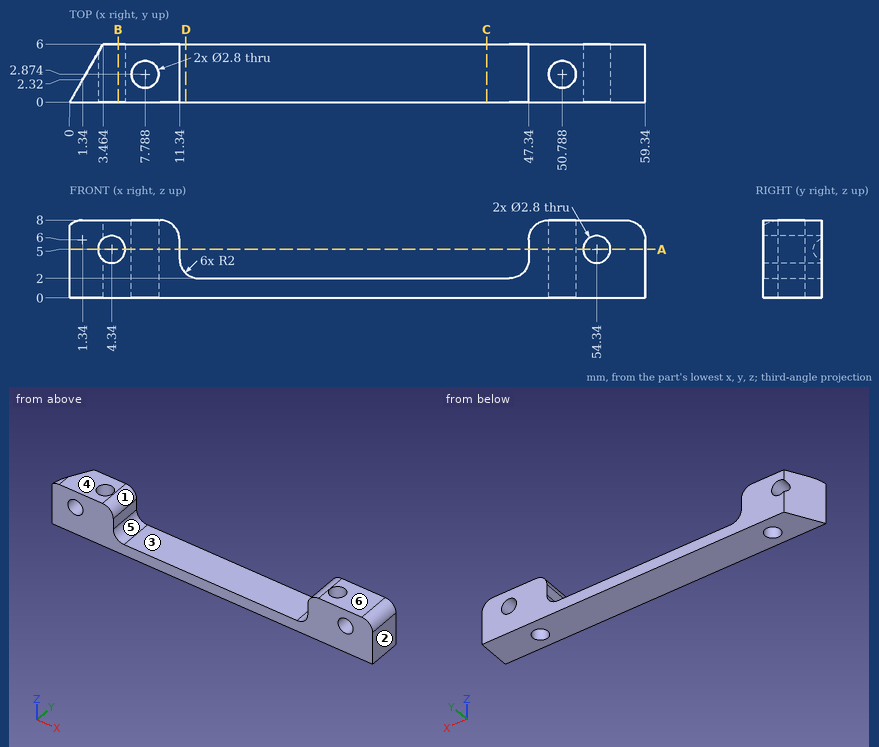
Design review of the part shown in the three views and the two pictorial views. Dimensions are in mm from the part's minimum x, y and z. A direction names the side the tool comes from. Round coordinates to 2 decimals unless told otherwise and drop trailing zeros. Loops run counter-clockwise (first coordinate to the right, second up) from the corner with the lowest first, then second, coordinate; pieces in that order, holes last. Notation, with made-up numbers: (-34, -32) -> (19, -32) arc R16 ccw to (19, -12) -> close; hole circle Ø6 at (73, 13.5). An arc over 180 degrees is marked (long way). Answer as a JSON object with one key per item and string values. Group by question number.
1) For line 1 (X direction, y = 3.5, z = 2.5) (1 decimal); line 2 (X direction, y = 2.75, z = 1) (1 decimal); line 3 (X direction, y = 3, z = 6.5) (1 decimal), list the stretches that pass through material, from the lowest coordinate up. Write a range as [from, to].
2) For pin 1 Ø2 at (x, y) = (21, 3) entering from -Z; pin 2 Ø2 at (x, y) = (7.79, 2.87) entering from -Z; pin 3 Ø2 at (y, z) = (2, 5.5) entering from -X; pin 4 Ø3 at (y, z) = (2, 7) entering from -X, all flat-tipped, find the tip position at first contact; note any pin that passes through.
3) We need section D-D on x = 12. Write out the cut boundary in (y, z) (1 decimal), then the cut area to 3 significant figures.
4) We need section C-C on x = 43. Write out the cut boundary in (y, z), then the cut area to 3 significant figures.
5) For the marked faces 5 and 6, list the 3-axis set-ups (+Z, -Z, +X, -X, +Y, -Y) from which the entire face can be reached by the end or side of a thin tool; tool diameter is ignored.
6) We need section A-A on z = 5. Write out the cut boundary in (x, y).
7) Mouldability with a two-part tool opening along X and no side actions: class the marked faces 1, 2, 3 and 4 as released by +X, released by -X, zero draft, split by the parting line, or undercut.
8) We need section B-B on x = 5. Write out the cut boundary in (y, z) (1 decimal), then the cut area to 3 significant figures.
Result set:
{
 "1": {"line 1": "[2, 6.5], [9, 12], [46.7, 49.5], [52, 59.3]", "line 2": "[1.6, 6.4], [9.2, 49.4], [52.2, 59.3]", "line 3": "[1.7, 6.4], [9.2, 11.3], [47.4, 49.4], [52.2, 59.3]"},
 "2": {"pin 1": "z = 0", "pin 2": "through", "pin 3": "x = 0.58", "pin 4": "x = 0.29"},
 "3": {"outline": "(0, 0) -> (6, 0) -> (6, 2.5) -> (0, 2.5) -> close", "area": "15.1 mm²"},
 "4": {"outline": "(0, 0) -> (6, 0) -> (6, 2) -> (0, 2) -> close", "area": "12.0 mm²"},
 "5": {"face 5": "+Z, +Y, -Y", "face 6": "+Z, +X, -X, +Y, -Y"},
 "6": {"outline": "(0, 0) -> (2.94, 0) -> (2.94, 5.09) -> close; (5.74, 0) -> (11.34, 0) -> (11.34, 6) -> (5.74, 6) -> close; (47.34, 0) -> (52.94, 0) -> (52.94, 6) -> (47.34, 6) -> close; (55.74, 0) -> (59.34, 0) -> (59.34, 6) -> (55.74, 6) -> close; hole circle Ø2.8 at (7.79, 2.87); hole circle Ø2.8 at (50.79, 2.87)"},
 "7": {"face 1": "undercut", "face 2": "released by +X", "face 3": "undercut", "face 4": "zero draft"},
 "8": {"outline": "(0, 0) -> (6, 0) -> (6, 3.8) -> (0, 3.8) -> close; (0, 6.2) -> (6, 6.2) -> (6, 8) -> (0, 8) -> close", "area": "33.2 mm²"}
}
